from build123d import *

# Parameters (mm, degrees)
SKETCH1_R             = 37.5
SKETCH1_R_2           = 34
BOSS_EXTRUDE1_DEPTH   = 35
BOSS_EXTRUDE2_START   = 15
SKETCH2_R             = 5
BOSS_EXTRUDE2_DEPTH   = 5
BOSS_EXTRUDE2_2_DEPTH = 5
BOSS_EXTRUDE3_START   = -15
SKETCH2_2_R           = 5
BOSS_EXTRUDE3_DEPTH   = 5
BOSS_EXTRUDE3_2_DEPTH = 5
BOSS_EXTRUDE4_DEPTH   = 70
BOSS_EXTRUDE5_START   = -70
BOSS_EXTRUDE5_DEPTH   = 70
SKETCH5_R             = 5.05
BOSS_EXTRUDE6_DEPTH   = 2.5
SKETCH6_W             = 0.149877485
SKETCH6_H             = 5
BOSS_EXTRUDE7_DEPTH   = 70


with BuildPart() as part:
    # Sketch1 → Boss-Extrude1 (new, symmetric)
    with BuildSketch(Plane(origin=(0, 0, 0), x_dir=(0, 0, -1), z_dir=(1, 0, 0))):
        Circle(SKETCH1_R)
        Circle(SKETCH1_R_2, mode=Mode.SUBTRACT)
    extrude(amount=BOSS_EXTRUDE1_DEPTH, both=True)



with BuildPart() as body_2:
    # Sketch2 → Boss-Extrude2 (new body)
    with BuildSketch(Plane.XY.offset(BOSS_EXTRUDE2_START)):
        with BuildLine():
            Line((-36.046360502, 95.880386994), (-35, 37.5))
            Line((-35, 37.5), (35, 37.5))
            Line((35, 37.5), (1.90425986, 105.037379634))
            ThreePointArc((1.90425986, 105.037379634), (-20.743145305, 115.677666176), (-36.046360502, 95.880386994))
        make_face()
        with Locations((-16.052783226, 96.238734902)):
            Circle(SKETCH2_R, mode=Mode.SUBTRACT)
    extrude(amount=BOSS_EXTRUDE2_DEPTH)


with BuildPart() as body_3:
    # Sketch2 → Boss-Extrude2 2 (new body)
    with BuildSketch(Plane.XY.offset(BOSS_EXTRUDE2_START)):
        with BuildLine():
            Line((-35, -37.5), (35, -37.5))
            Line((35, -37.5), (28.89703955, -106.961265098))
            ThreePointArc((28.89703955, -106.961265098), (12.060917272, -126.709426475), (-10.101948226, -113.209341881))
            Line((-10.101948226, -113.209341881), (-35, -37.5))
        make_face()
        with Locations((8.89703955, -106.961265098)):
            Circle(SKETCH2_R, mode=Mode.SUBTRACT)
    extrude(amount=BOSS_EXTRUDE2_2_DEPTH)


with BuildPart() as body_4:
    # Sketch2<2> → Boss-Extrude3 (new body)
    with BuildSketch(Plane.XY.offset(BOSS_EXTRUDE3_START)):
        with BuildLine():
            Line((-36.046360502, 95.880386994), (-35, 37.5))
            Line((-35, 37.5), (35, 37.5))
            Line((35, 37.5), (1.90425986, 105.037379634))
            ThreePointArc((1.90425986, 105.037379634), (-20.743145305, 115.677666176), (-36.046360502, 95.880386994))
        make_face()
        with Locations((-16.052783226, 96.238734902)):
            Circle(SKETCH2_2_R, mode=Mode.SUBTRACT)
    extrude(amount=BOSS_EXTRUDE3_DEPTH)


with BuildPart() as body_5:
    # Sketch2<2> → Boss-Extrude3 2 (new body)
    with BuildSketch(Plane.XY.offset(BOSS_EXTRUDE3_START)):
        with BuildLine():
            Line((-35, -37.5), (35, -37.5))
            Line((35, -37.5), (28.89703955, -106.961265098))
            ThreePointArc((28.89703955, -106.961265098), (12.060917272, -126.709426475), (-10.101948226, -113.209341881))
            Line((-10.101948226, -113.209341881), (-35, -37.5))
        make_face()
        with Locations((8.89703955, -106.961265098)):
            Circle(SKETCH2_2_R, mode=Mode.SUBTRACT)
    extrude(amount=BOSS_EXTRUDE3_2_DEPTH)


with BuildPart() as part_1:
    add(part.part)

    add(body_2.part)  # Boss-Extrude4 merges body 2

    add(body_4.part)  # Boss-Extrude4 merges body 4
    # Sketch3 → Boss-Extrude4 (add)
    with BuildSketch(Plane(origin=(35, 0, 0), x_dir=(0, 0, -1), z_dir=(1, 0, 0))):
        with BuildLine():
            Line((-20, 37.5), (-20, 31.721443851))
            ThreePointArc((-20, 31.721443851), (-2.828923646, 37.393143636), (15, 34.369317712))
            Line((15, 34.369317712), (15, 37.5))
            Line((15, 37.5), (15, 38.756727822))
            Line((15, 38.756727822), (-20, 38.756727822))
            Line((-20, 38.756727822), (-20, 37.5))
        make_face()
    extrude(amount=-BOSS_EXTRUDE4_DEPTH)


    add(body_3.part)  # Boss-Extrude5 merges body 3

    add(body_5.part)  # Boss-Extrude5 merges body 5
    # Sketch4 → Boss-Extrude5 (add)
    with BuildSketch(Plane.ZY.offset(35).offset(BOSS_EXTRUDE5_START)):
        with BuildLine():
            Line((-15, -39.232593617), (20, -39.232593617))
            Line((20, -39.232593617), (20, -31.721443851))
            ThreePointArc((20, -31.721443851), (2.828923646, -37.393143636), (-15, -34.369317712))
            Line((-15, -34.369317712), (-15, -39.232593617))
        make_face()
    extrude(amount=BOSS_EXTRUDE5_DEPTH)



with BuildPart() as body_2_2:
    # Sketch5 → Boss-Extrude6 (new, symmetric)
    with BuildSketch(Plane(origin=(0, 0, 0), x_dir=(1, 0, 0), z_dir=(0, 1, 0))):
        with BuildLine():
            Line((35, 37.5), (-35, 37.5))
            Line((-35, 37.5), (-35.078450863, 37.500626944))
            Line((-35.078450863, 37.500626944), (13.155155891, 89.33933901))
            ThreePointArc((13.155155891, 89.33933901), (28.276948524, 89.13371958), (35.534104179, 75.865540218))
            Line((35.534104179, 75.865540218), (35, 37.5))
        make_face()
        with Locations(Location((20.539917261, 76.283102971, 0), (0, 0, 270))):
            Circle(SKETCH5_R, mode=Mode.SUBTRACT)
    extrude(amount=BOSS_EXTRUDE6_DEPTH, both=True)


with BuildPart() as part_2:
    add(part_1.part)

    add(body_2_2.part)  # Boss-Extrude7 merges body 2 2
    # Sketch6 → Boss-Extrude7 (add)
    with BuildSketch(Plane(origin=(35, 0, 0), x_dir=(0, 0, -1), z_dir=(1, 0, 0))):
        with Locations((37.425061258, 0)):
            Rectangle(SKETCH6_W, SKETCH6_H)
    extrude(amount=-BOSS_EXTRUDE7_DEPTH)


solid = part_2.part
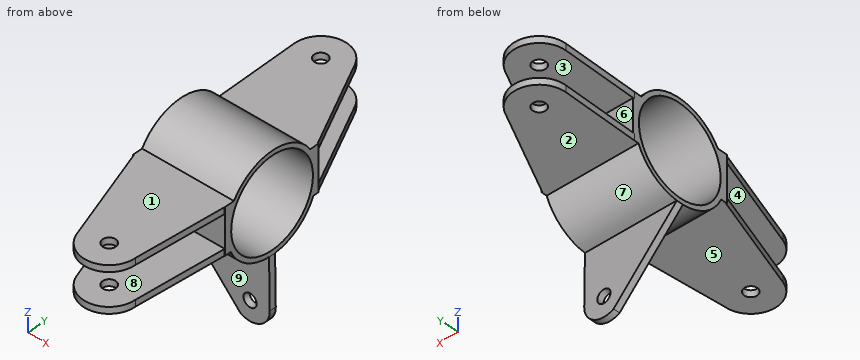
Read the model definition and answer for the solid it produces. Units are mm, in the model's axes. Face numbers are marked on the shaded views. A direction names the side the tool comes from. Round coordinates to 2 decimals unless told otherwise and drop trailing zeros. Write each loop counter-clockwise with the first axis right and the second up, starting at its lowest first coordinate (ties: lowest second). Pieces come first, ordered by that corner, then holes. Notation, with made-up numbers: M 63.25,0.5 L 85.25,0.5 A12 cw 85.25,22.5 Z; hole C -17.5,-10 d3. An arc over 180 degrees is marked long. Use a Markdown table: item, result.
1) Straight lines are drawn through the part: line 1 along Z through (x, y) = (-15, -92); line 2 along Y through (x, z) = (2, 1.5); line 3 along Y through (x, z) = (-2.5, -57). For each, find the intervals that lie inside material, in ascending order. Write a range as [from, to].
Answers follow:
| item | result |
|---|---|
| line 1 | z = [-15, -10], [15, 20] |
| line 2 | y = [-39.23, -33.97], [33.97, 38.76] |
| line 3 | y = [-2.5, 2.5] |
2) Flat-ended cylindrical pins translate along their axes: pin 1 (21 mm diameter, centred on x = -13.5, y = -98, fed in from +Z); pin 2 (6 mm diameter, centred on x = 23.5, z = -41.5, fed in from +Y); pin 3 (17.5 mm diameter, centred on x = -1.5, z = 2, fed in from +Y). Find the tip coordinate at first contact, or state that the pin passes through.
Answers follow:
| item | result |
|---|---|
| pin 1 | stops at z = 20 |
| pin 2 | stops at y = 2.5 |
| pin 3 | stops at y = 38.76 |
3) For a pull along Z with two mould halves and no side action, classify the marked faces 6, 7, 8 and 9 as pulls with the +Z half, pulls with the -Z half, needs draft (parallel to the pull), parting line crosses it, or undercut.
Answers follow:
| item | result |
|---|---|
| face 6 | undercut |
| face 7 | pulls with the -Z half |
| face 8 | undercut |
| face 9 | needs draft |
4) A tool of negligible diameter and unlimited length cuts with its end or side. For the marked faces 1, 2, 3, 4 and 5, from which of +Z, -Z, +X, -X, +Y, -Y can it reach the whole face along a straight path? Write none if from no direction.
Answers follow:
| item | result |
|---|---|
| face 1 | +Z, +X, -X, -Y |
| face 2 | -Z, +X, -X, +Y |
| face 3 | +X, -X, +Y |
| face 4 | +X, -X, -Y |
| face 5 | -Z, +X, -X, -Y |
5) The part is cut by section C-C (x = 18). Write down the section's boundary in (y, z), plus the area to 3 significant figures.
Answers follow:
| item | result |
|---|---|
| outline | M -124.77,-15 L -34.37,-15 A37.5 ccw -2.5,-37.42 L -2.5,-71.92 L 2.5,-71.92 L 2.5,-37.42 A37.5 ccw 34.37,-15 L 72.19,-15 L 72.19,-10 L 38.76,-10 L 38.76,15 L 72.19,15 L 72.19,20 L 31.72,20 A37.5 ccw -31.72,20 L -124.77,20 L -124.77,15 L -39.23,15 L -39.23,-10 L -124.77,-10 Z; M -2.5,-91.07 L 2.5,-91.07 L 2.5,-80.65 L -2.5,-80.65 Z; hole C 0,0 d68 |
| area | 2,410 mm2 |
6) The part is cut by section B-B (z = 0). Write down the section's boundary in (x, y), plus the area to 3 significant figures.
Answers follow:
| item | result |
|---|---|
| outline | M -35,-39.23 L 35,-39.23 L 35,-34 L -35,-34 Z; M -35,34 L 35,34 L 35,38.76 L -35,38.76 Z |
| area | 699 mm2 |
7) The part is cut by section D-D (y = 22.5). Write down the section's boundary in (x, z).
Answers follow:
| item | result |
|---|---|
| outline | M -35,-30 L 35,-30 L 35,-25.49 L -35,-25.49 Z; M -35,25.49 L 35,25.49 L 35,30 L -35,30 Z |
8) The part is cut by section A-A (x = -15). Give the number of separate pieces and of enclosed holes in the cut face, plus the area to 3 significant figures.
Answers follow:
| item | result |
|---|---|
| separate pieces | 3 |
| enclosed holes | 1 |
| area | 2,370 mm2 |
